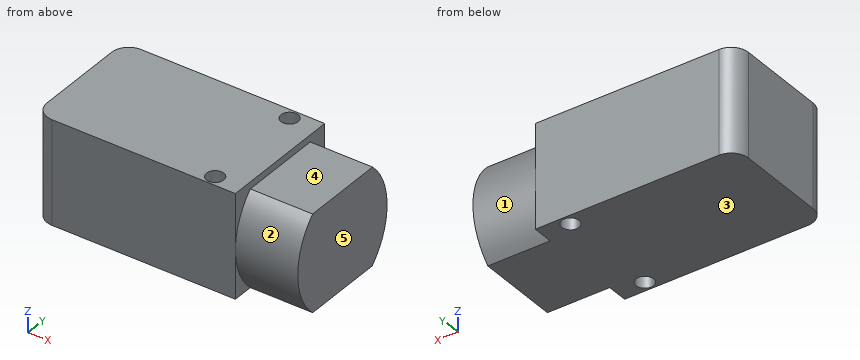
Autodesk Inventor part; units mm, degrees
ref_plane "YZ Plane" through (0, 0, 0) normal (1, 0, 0) x (0, 1, 0)
ref_plane "XZ Plane" through (0, 0, 0) normal (0, 1, 0) x (-1, 0, 0)
ref_plane "XY Plane" through (0, 0, 0) normal (0, 0, 1) x (1, 0, 0)
sketch "Sketch1" plane through (0, 0, 0) normal (0, 0, 1) x (1, 0, 0)
  line L0 (0, 0) -> (36.83, 0)
  line L1 (36.83, 0) -> (36.83, -22.86)
  line L2 (36.83, -22.86) -> (0, -22.86)
  line L3 (0, -22.86) -> (0, 0)
  dimension "d0" = 36.83
  dimension "d1" = 22.86
extrude "Extrusion1" add sketch "Sketch1" along normal blind 19.05
fillet "Fillet1" radius 3.175 2 edges at (0, 0, 9.525) (0, -22.86, 9.525)
sketch "Sketch2" plane through (36.83, -22.86, 0) normal (1, 0, 0) x (0, 0, -1)
  line L0 (0, 22.86) -> (-19.05, 22.86)
  line L1 (0, 0) -> (-19.05, 0)
  line L2 (-19.05, 0) -> (-19.05, 22.86)
  arc A0 (0, 19.05) -> (-17.78, 19.1328) centre (-8.93, 10.4897) ccw
  arc A1 (-17.78, 3.81) -> (0, 3.81) centre (-8.89, 12.2767) ccw
  line L3 (0, 19.05) -> (0, 3.81)
  line L4 (0, 22.86) -> (0, 0)
  line L5 (-19.05, 3.175) -> (0, 3.175)
  line L6 (-17.78, 3.81) -> (-17.78, 19.1328)
  dimension "d5" = 3.81
  dimension "d6" = 3.81
  dimension "d7" = 1.27
  dimension "d8" = 1.27
extrude "Extrusion2" add sketch "Sketch2" along normal blind 11.43 contours A0 L3 A1 L5 L6 | A1 L5
sketch "Sketch3" plane through (0, 0, 19.05) normal (0, 0, 1) x (1, 0, 0)
  circle A0 centre (31.75, -1.905) radius 1.5875
  line L0 (36.83, -22.86) -> (36.83, 0)
  line L1 (36.83, 0) -> (3.175, 0)
  circle A1 centre (31.75, -20.955) radius 1.5875
  line L2 (3.175, -22.86) -> (36.83, -22.86)
  point P0 (0, 0)
  dimension "d11" = 3.175
  dimension "d12" = 5.08
  dimension "d13" = 1.905
  dimension "d14" = 1.905
  dimension "d15" = 3.175
extrude "Extrusion3" cut sketch "Sketch3" against normal blind 25.4
properties part number "MotorFrame" material "ABS Plastic"
Design review of the part built by this model. Coordinates are the model's own, in mm. Face numbers are marked on the shaded views. A direction names the side the tool comes from. Give positions to 0.01 mm unless a question says otherwise; leave off trailing zeros. Loops run counter-clockwise (first coordinate to the right, second up) from the corner with the lowest first, then second, coordinate; pieces in that order, holes last. Notation, with made-up numbers: (-35, 60.5) -> (-12, 60.5) arc R17 cw to (-12, 65.5) -> close; hole circle Ø11 at (-5.5, 47). An arc over 180 degrees is marked (long way). One line per item, written item: value.
Q1. For L1, parallel to Y at x = 31.75, z = 7.5; L2, parallel to Y at x = 33, z = 10; L3, parallel to Y at x = 40, z = 9.25, list the stretches that pass through material, from the lowest coordinate up.
Numbers:
L1: y = -22.86 to -22.54, -19.37 to -3.49, -0.32 to 0
L2: y = -22.86 to -21.93, -19.98 to -2.88, -0.93 to 0
L3: y = -22.85 to 0
Q2. Machinability: for the marked faces 1, 2, 3, 4 and 5, which of the approach directions +Z, -Z, +X, -X, +Y, -Y give a long, thin tool a straight path to every point of the face, cutting with its end or side? Answer none if there is none.
Numbers:
face 1: +X, +Y
face 2: +X, -Y
face 3: -Z, +X, -X, +Y, -Y
face 4: +Z, +X, +Y, -Y
face 5: +Z, -Z, +X, +Y, -Y
Q3. We need section C-C on y = -4.5. Give the boundary of the cut face in (x, z), and give its area (3 significant figures).
Numbers:
outline: (0, 0) -> (48.26, 0) -> (48.26, 17.78) -> (36.83, 17.78) -> (36.83, 19.05) -> (0, 19.05) -> close
area: 905 mm^2
Q4. We need section B-B on z = 8.25. Give the number of separate pieces and of enclosed holes in the cut face, and give its area (3 significant figures).
Numbers:
separate pieces: 1
enclosed holes: 2
area: 1,080 mm^2
Q5. We need section A-A on x = 31.75. Give the boundary of the cut face in (y, z).
Numbers:
outline: (-22.86, 0) -> (-22.54, 0) -> (-22.54, 19.05) -> (-22.86, 19.05) -> close; (-19.37, 0) -> (-3.49, 0) -> (-3.49, 19.05) -> (-19.37, 19.05) -> close; (-0.32, 0) -> (0, 0) -> (0, 19.05) -> (-0.32, 19.05) -> close
